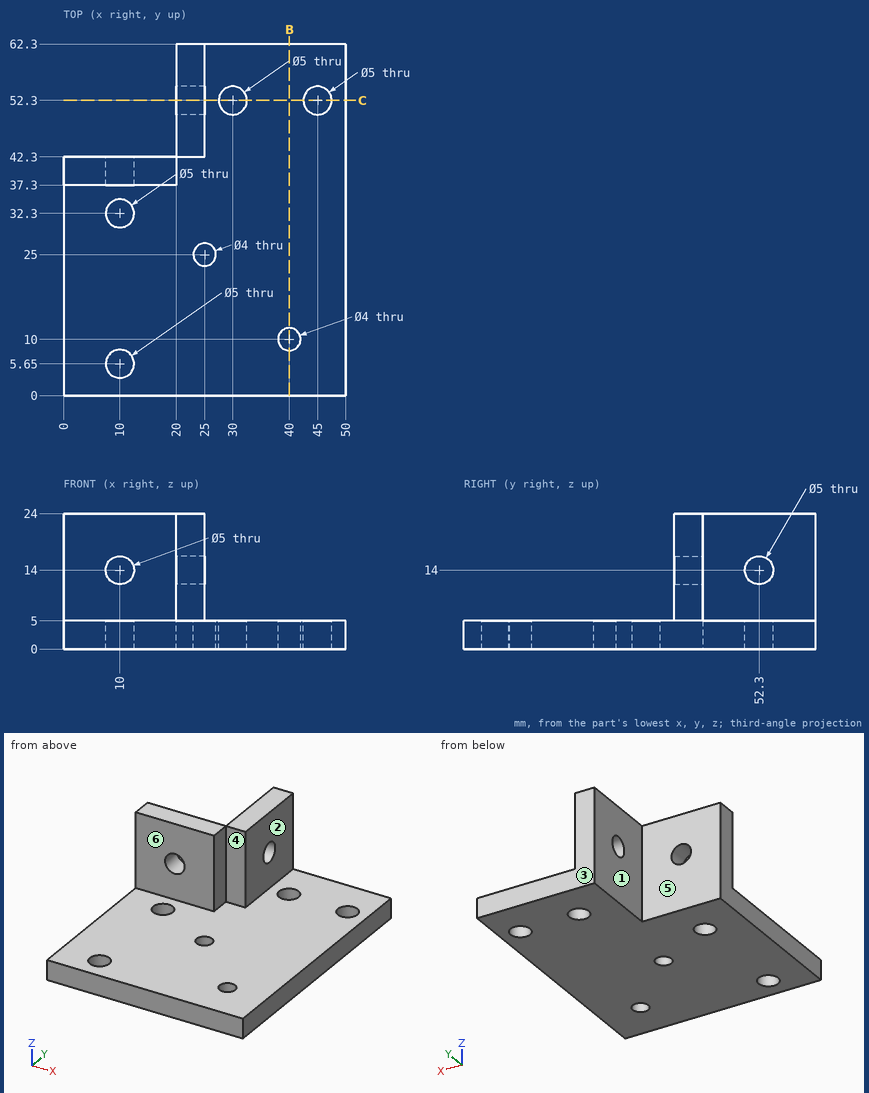
Check sheet for the drawn part. Datum: minimum x, y, z corner. Units: mm. A direction names the side the tool comes from. Round coordinates to 2 decimals unless told otherwise and drop trailing zeros. Order: outer loops, then holes, each group sorted by start corner. A loop starts at its lowest first (then second) coordinate and runs counter-clockwise, first axis right, second up. Notation, with made-up numbers: M -35,88.5 L -7,88.5 A25 cw -7,127.5 Z; hole C 64.5,-30.5 d9. An arc over 180 degrees is marked long. Answer in a Markdown table with one row per item.
(1) Material ranges on line 1 along Y through (x, z) = (10, 1.7); line 2 along X through (y, z) = (52.3, 3.45); line 3 along X through (y, z) = (5.65, 3.4), recorded low to high. Write a range as from..to.
Findings:
| item | result |
|---|---|
| line 1 | y = 0..3.15, 8.15..29.8, 34.8..42.3 |
| line 2 | x = 20..27.5, 32.5..42.5, 47.5..50 |
| line 3 | x = 0..7.5, 12.5..50 |
(2) Section check B-B on x = 40. Record the boundary of the cut face in (y, z), plus the area to 4 significant figures.
Findings:
| item | result |
|---|---|
| outline | M 0,0 L 8,0 L 8,5 L 0,5 Z; M 12,0 L 62.3,0 L 62.3,5 L 12,5 Z |
| area | 291.5 mm^2 |
(3) Gauge pin test, flat ends, axial feed: pin 1 (2.5 mm diameter, centred on x = 23.5, z = 13.5, fed in from -Y); pin 2 (6.5 mm diameter, centred on x = 25, y = 25, fed in from -Z); pin 3 (1 mm diameter, centred on x = 18.5, y = 11, fed in from +Z); pin 4 (2.5 mm diameter, centred on y = 41, z = 11, fed in from +X). Record the tip position at first contact, or that the pin passes through.
Findings:
| item | result |
|---|---|
| pin 1 | stops at y = 42.3 |
| pin 2 | stops at z = 0 |
| pin 3 | stops at z = 5 |
| pin 4 | stops at x = 20 |
(4) Draft check along X on the marked faces 1, 2 and 3. Enter one of: +X half, -X half, draft (parallel to the pull), parting line (faces both ways), or undercut.
Findings:
| item | result |
|---|---|
| face 1 | -X half |
| face 2 | +X half |
| face 3 | draft |
(5) Section check C-C on y = 52.3. Record the boundary of the cut face in (x, z), plus the area to 3 significant figures.
Findings:
| item | result |
|---|---|
| outline | M 20,0 L 27.5,0 L 27.5,5 L 25,5 L 25,11.5 L 20,11.5 Z; M 20,16.5 L 25,16.5 L 25,24 L 20,24 Z; M 32.5,0 L 42.5,0 L 42.5,5 L 32.5,5 Z; M 47.5,0 L 50,0 L 50,5 L 47.5,5 Z |
| area | 170 mm^2 |
(6) Set-up check for the marked faces 4, 5 and 6: record each of +Z, -Z, +X, -X, +Y, -Y from which the full face is reachable in a straight line by a thin tool's end or side.
Findings:
| item | result |
|---|---|
| face 4 | +Z, +X, -Y |
| face 5 | +Z, -Z, -X, +Y |
| face 6 | +Z, +X, -X, -Y |
